Autodesk Inventor part; units mm, degrees
ref_plane "YZ Plane" through (0, 0, 0) normal (1, 0, 0) x (0, 1, 0)
ref_plane "XZ Plane" through (0, 0, 0) normal (0, 1, 0) x (-1, 0, 0)
ref_plane "XY Plane" through (0, 0, 0) normal (0, 0, 1) x (1, 0, 0)
sketch "Skizze1" plane through (0, 0, 0) normal (0, 0, 1) x (1, 0, 0)
  circle A0 centre (16.76, 0) radius 1.25
  circle A1 centre (-16.76, 0) radius 1.25
  line L0 (-6.25, 16) -> (-11.9414, 16)
  line L1 (-2.25, 20) -> (-6.25, 16)
  line L2 (2.25, 20) -> (-2.25, 20)
  line L3 (6.25, 16) -> (2.25, 20)
  line L4 (11.9414, 16) -> (6.25, 16)
  line L5 (11.9414, 16) -> (12.9414, 15)
  line L6 (12.9414, -15) -> (12.9414, 15)
  line L7 (11.9414, -16) -> (12.9414, -15)
  line L8 (-11.9414, -16) -> (11.9414, -16)
  line L9 (-11.9414, -16) -> (-12.9414, -15)
  line L10 (-12.9414, 15) -> (-12.9414, -15)
  line L11 (-12.9414, 15) -> (-11.9414, 16)
  circle A2 centre (0, 0) radius 20.5786
  point P0 (0, 0)
extrude "Extrusion1" add sketch "Skizze1" along normal blind 2 contours L1 L2 L3 L4 L5 L6 L7 L8 L9 L10 L11 L0 | A2
sketch "Skizze2" plane through (0, 0, 2) normal (0, 0, 1) x (1, 0, 0)
  point P0 (0, 0)
sketch "Skizze3" plane through (0, 0, 2) normal (0, 0, 1) x (1, 0, 0)
  line L0 (-12.1, -11.9394) -> (-9.9, -11.9394)
  line L1 (-9.9, -11.9394) -> (-9.9, 11.9394)
  line L2 (-9.9, 11.9394) -> (-12.1, 11.9394)
  line L3 (-12.1, 11.9394) -> (-12.1, -11.9394)
  line L4 (-7.7, 14.502) -> (-5.5, 14.502)
  line L5 (-5.5, 14.502) -> (-5.5, -14.502)
  line L6 (-5.5, -14.502) -> (-7.7, -14.502)
  line L7 (-7.7, -14.502) -> (-7.7, 14.502)
  line L8 (-3.3, 15.4709) -> (-1.1, 15.4709)
  line L9 (-1.1, 15.4709) -> (-1.1, -15.4709)
  line L10 (-1.1, -15.4709) -> (-3.3, -15.4709)
  line L11 (-3.3, -15.4709) -> (-3.3, 15.4709)
  circle A0 centre (-16.76, 0) radius 1.25
  circle A1 centre (16.76, 0) radius 1.25
  circle A2 centre (0, 0) radius 20.5786
  line L12 (-16.76, 0) -> (0, 0) construction
  circle A3 centre (0, 0) radius 15.51 construction
  line L13 (0, 0) -> (0, 15.51)
  point P0 (0, 0)
  dimension "d2" = 2.2
  dimension "d3" = 2.2
  dimension "d4" = 2.2
  dimension "d5" = 2.2
  dimension "d6" = 2.2
  dimension "d7" = 1.1
ref_plane "Arbeitsebene1" through (0, 0, 2) normal (1, 0, 0) x (0, 1, 0)
extrude "Extrusion2" cut sketch "Skizze3" against normal through all contours L3 L2 L1 L0 | L4 L5 L6 L7 | L8 L9 L10 L11
mirror "Spiegeln1" about plane through (0, 0, 2) normal (1, 0, 0) of "Extrusion2"
sketch "Skizze4" plane through (0, 0, 2) normal (0, 0, 1) x (1, 0, 0)
  line L0 (5.5, -14.502) -> (5.5, 14.502)
  line L1 (5.5, 14.502) -> (7.7, 14.502)
  line L2 (7.7, 14.502) -> (7.7, -14.502)
  line L3 (7.7, -14.502) -> (5.5, -14.502)
  line L4 (1.1, -15.4709) -> (1.1, 15.4709)
  line L5 (1.1, 15.4709) -> (3.3, 15.4709)
  line L6 (3.3, 15.4709) -> (3.3, -15.4709)
  line L7 (3.3, -15.4709) -> (1.1, -15.4709)
  line L8 (9.9, 11.9394) -> (12.1, 11.9394)
  line L9 (12.1, 11.9394) -> (12.1, -11.9394)
  line L10 (12.1, -11.9394) -> (9.9, -11.9394)
  line L11 (9.9, -11.9394) -> (9.9, 11.9394)
  line L12 (-7.7, -14.502) -> (-7.7, 14.502)
  line L13 (-7.7, 14.502) -> (-5.5, 14.502)
  line L14 (-5.5, 14.502) -> (-5.5, -14.502)
  line L15 (-5.5, -14.502) -> (-7.7, -14.502)
  line L16 (-9.9, 11.9394) -> (-9.9, -11.9394)
  line L17 (-9.9, -11.9394) -> (-12.1, -11.9394)
  line L18 (-12.1, -11.9394) -> (-12.1, 11.9394)
  line L19 (-12.1, 11.9394) -> (-9.9, 11.9394)
  line L20 (-3.3, -15.4709) -> (-3.3, 15.4709)
  line L21 (-3.3, 15.4709) -> (-1.1, 15.4709)
  line L22 (-1.1, 15.4709) -> (-1.1, -15.4709)
  line L23 (-1.1, -15.4709) -> (-3.3, -15.4709)
  circle A0 centre (-16.76, 0) radius 1.25
  circle A1 centre (16.76, 0) radius 1.25
  circle A2 centre (0, 0) radius 20.5786
  point P0 (0, 0)
hole "Bohrung1" at (-16.76, 0, 2) at (16.76, 0, 2) direction (0, 0, -1) diameter 3.2 end through all
equation "\"d3\" = d2"
equation "\"d4\" = d3"
equation "\"d5\" = d4"
equation "\"d6\" = d3"
equation "\"d7\" = 0.5 * d2"
properties part number "Wrist_Cover" material "ABS-Kunststoff"
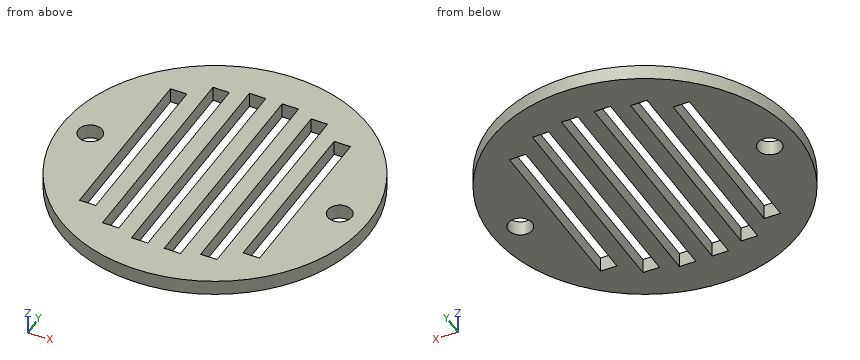
Part model, mm, in its own coordinate system. Give positions to 0.01 mm unless a question says otherwise; leave off trailing zeros. Write each loop counter-clockwise with the first axis right and the second up, starting at its lowest first coordinate (ties: lowest second). Pieces come first, ordered by that corner, then holes. Notation, with made-up numbers: M -28,58.5 L 8,58.5 A35 cw 8,96.5 Z; hole C -14.75,50 d4. An arc over 180 degrees is marked long. Use CSV: the item, a comma, the result in double quotes.
Item 1: Slice it at B-B on z = 1.7. State how many separate pieces and enclosed holes the cut face has, plus the area to 3 significant figures.
Taken from the geometry:
separate pieces,"1"
enclosed holes,"8"
area,"945 mm²"
Item 2: Slice it at C-C on y = 10.5. Write the cut outline in (x, z), plus the area to 3 significant figures.
Taken from the geometry:
outline,"M -17.7,0 L -12.1,0 L -12.1,2 L -17.7,2 Z; M -9.9,0 L -7.7,0 L -7.7,2 L -9.9,2 Z; M -5.5,0 L -3.3,0 L -3.3,2 L -5.5,2 Z; M -1.1,0 L 1.1,0 L 1.1,2 L -1.1,2 Z; M 3.3,0 L 5.5,0 L 5.5,2 L 3.3,2 Z; M 7.7,0 L 9.9,0 L 9.9,2 L 7.7,2 Z; M 12.1,0 L 17.7,0 L 17.7,2 L 12.1,2 Z"
area,"44.4 mm²"
Item 3: Pin check, flat tips, straight feed: P1, Ø1, axis at x = 11.5, z = 1, coming from the +Y side; P2, Ø1, axis at y = 15, z = 1.5, coming from the +X side; P3, Ø1, axis at x = -2.5, z = 1, coming from the +Y side. Stop position of each tip, or through.
Taken from the geometry:
P1,"stops at y = 17.39"
P2,"stops at x = 14.6"
P3,"stops at y = 20.48"
Item 4: Slice it at A-A on x = -11. Write the cut outline in (y, z).
Taken from the geometry:
outline,"M -17.39,0 L -11.94,0 L -11.94,2 L -17.39,2 Z; M 11.94,0 L 17.39,0 L 17.39,2 L 11.94,2 Z"
Item 5: Drill centre lines: probe 1 along Y at (x, z) = (-16.76, 1.3); probe 2 along X at (y, z) = (15, 1.45); probe 3 along X at (y, z) = (12, 1.1). Where is each one in solid material? Low to high.
Taken from the geometry:
probe 1,"y = -11.94 to -1.6, 1.6 to 11.94"
probe 2,"x = -14.09 to -3.3, -1.1 to 1.1, 3.3 to 14.09"
probe 3,"x = -16.72 to -7.7, -5.5 to -3.3, -1.1 to 1.1, 3.3 to 5.5, 7.7 to 16.72"
